Geometry: see drawing. Coordinates: mm, zero at the bounding-box minimum. Coordinates: 2 decimals unless noted, no trailing zeros. Loops run counter-clockwise (first coordinate to the right, second up) from the corner with the lowest first, then second, coordinate; pieces in that order, holes last. Notation, with made-up numbers: (-35, -23) - (-11, -23) arc R21 cw to (-11, 6) - close; hole circle Ø5 at (38.5, 29.5). An arc over 180 degrees is marked (long way). Write item = value, one per line. Start each with the question number.
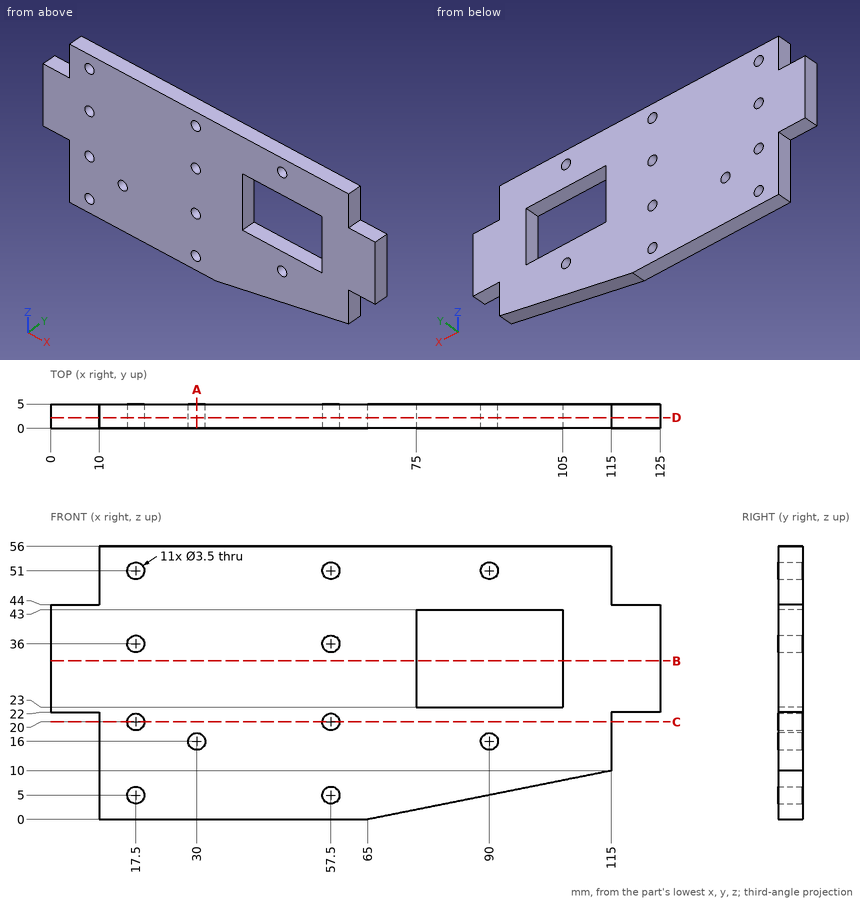
Item 1: Cut plane C-C (z = 20). Return the cut outline in (x, y).
Item 2: Cut plane A-A (x = 30). Return the cut outline in (y, z).
Item 3: Cut plane B-B (z = 32.5). Return the cut outline in (x, y).
Item 4: Cut plane D-D (y = 2.2). State how many separate pieces and enclosed holes the cut face has, then the cut area to 3 significant figures.
Item 5: Material intervals for L1, parallel to X at y = 1.5, z = 16; L2, parallel to X at y = 0.45, z = 51; L3, parallel to X at y = 3.4, z = 26.5, sorted ascending. Write a range as [from, to].
Item 6: First-contact query: pin 1 (3 mm diameter, centred on x = 57.5, z = 5, fed in from -Y). Flat tip, straight axial feed; report the tip coordinate or a pass-through.
Responses:
q1.outline = (10, 0) - (15.75, 0) - (15.75, 5) - (10, 5) - close; (19.25, 0) - (55.75, 0) - (55.75, 5) - (19.25, 5) - close; (59.25, 0) - (115, 0) - (115, 5) - (59.25, 5) - close
q2.outline = (0, 0) - (5, 0) - (5, 14.25) - (0, 14.25) - close; (0, 17.75) - (5, 17.75) - (5, 56) - (0, 56) - close
q3.outline = (0, 0) - (75, 0) - (75, 5) - (0, 5) - close; (105, 0) - (125, 0) - (125, 5) - (105, 5) - close
q4.separate_pieces = 1
q4.enclosed_holes = 12
q4.area = 5,360 mm2
q5.L1 = [10, 28.25], [31.75, 88.25], [91.75, 115]
q5.L2 = [10, 15.75], [19.25, 55.75], [59.25, 88.25], [91.75, 115]
q5.L3 = [0, 75], [105, 125]
q6.pin_1 = through
